Check sheet for the modelled part. Datum: model origin and axes. Units: mm. A direction names the side the tool comes from. Round coordinates to 2 decimals unless told otherwise and drop trailing zeros. Write each loop counter-clockwise with the first axis right and the second up, starting at its lowest first coordinate (ties: lowest second). Pieces come first, ordered by that corner, then holes. Notation, with made-up numbers: (29, 5.5) -> (78, 5.5) arc R16 cw to (78, 22.5) -> close; hole circle Ø3 at (71, 62). An arc over 180 degrees is marked (long way). Write item = value, one per line.
from build123d import *

# Parameters (mm, degrees)
SKETCH2_W                      = 50
SKETCH2_H                      = 50
BOSS_EXTRUDE1_DEPTH            = 10
SKETCH3_W                      = 9
SKETCH3_H                      = 9
CUT_EXTRUDE1_DEPTH             = 10
SKETCH4_R                      = 23.125
CUT_EXTRUDE2_DEPTH             = 2.5
F_4_0MM_DOWEL_HOLE1_D          = 4
FILLET1_R                      = 1
FILLET2_R                      = 10
CUT_EXTRUDE3_DEPTH             = 2.5
CBORE_FOR_M3_SHCS2_D           = 3.4
CBORE_FOR_M3_SHCS2_CBORE_D     = 6.5
CBORE_FOR_M3_SHCS2_CBORE_DEPTH = 3
SKETCH21_R                     = 3.25
CUT_EXTRUDE5_DEPTH             = 2.5
BOSS_EXTRUDE2_DEPTH            = 8
CHAMFER1_SIZE                  = 0.5


with BuildPart() as part:
    # Sketch2 → Boss-Extrude1 (new body)
    with BuildSketch(Plane(origin=(0, 0, 0), x_dir=(1, 0, 0), z_dir=(0, 1, 0))):
        Rectangle(SKETCH2_W, SKETCH2_H)
    extrude(amount=BOSS_EXTRUDE1_DEPTH)

    # Sketch3 → Cut-Extrude1 (cut)
    with BuildSketch(Plane(origin=(0, 10, 0), x_dir=(1, 0, 0), z_dir=(0, 1, 0))):
        Rectangle(SKETCH3_W, SKETCH3_H)
    extrude(amount=-CUT_EXTRUDE1_DEPTH, mode=Mode.SUBTRACT)

    # Sketch4 → Cut-Extrude2 (cut)
    with BuildSketch(Plane.XZ):
        Circle(SKETCH4_R)
    extrude(amount=-CUT_EXTRUDE2_DEPTH, mode=Mode.SUBTRACT)

    # Ø4.0mm Dowel Hole1 (through all)
    with Locations(Plane(origin=(0, 10, 0), x_dir=(1, 0, 0), z_dir=(0, 1, 0))):
        with Locations((-9, 5.5), (9, 5.5), (9, -5.5), (-9, -5.5)):
            Hole(F_4_0MM_DOWEL_HOLE1_D / 2)

    # Fillet1
    fillet1_edges = [part.edges().sort_by_distance(p)[0] for p in [
        (4.5, 6.25, -4.5),
        (-4.5, 6.25, -4.5),
        (-4.5, 6.25, 4.5),
        (4.5, 6.25, 4.5),
    ]]
    fillet(fillet1_edges, radius=FILLET1_R)

    # Fillet2
    fillet2_edges = [part.edges().sort_by_distance(p)[0] for p in [
        (-25, 5, -25),
        (25, 5, -25),
        (25, 5, 25),
        (-25, 5, 25),
    ]]
    fillet(fillet2_edges, radius=FILLET2_R)

    # Sketch17 → Cut-Extrude3 (cut)
    with BuildSketch(Plane(origin=(0, 10, 0), x_dir=(1, 0, 0), z_dir=(0, 1, 0))):
        with BuildLine():
            Line((5, 7.75), (11.25, 7.75))
            Line((11.25, 7.75), (11.25, -20.75))
            Line((11.25, -20.75), (-11.25, -20.75))
            Line((-11.25, -20.75), (-11.25, 7.75))
            Line((-11.25, 7.75), (-5, 7.75))
            ThreePointArc((-5, 7.75), (0, 12.75), (5, 7.75))
        make_face()
    extrude(amount=-CUT_EXTRUDE3_DEPTH, mode=Mode.SUBTRACT)

    # CBORE for M3 SHCS2 (through all)
    with Locations(Plane(origin=(0, 7.5, 0), x_dir=(1, 0, 0), z_dir=(0, 1, 0))):
        with Locations((0, -9), (0, 9)):
            CounterBoreHole(CBORE_FOR_M3_SHCS2_D / 2, CBORE_FOR_M3_SHCS2_CBORE_D / 2, CBORE_FOR_M3_SHCS2_CBORE_DEPTH)

    # Sketch21 → Cut-Extrude5 (cut)
    with BuildSketch(Plane(origin=(0, 10, 0), x_dir=(1, 0, 0), z_dir=(0, 1, 0))):
        with Locations((-9, 5.5)):
            Circle(SKETCH21_R)
        with Locations((9, 5.5)):
            Circle(SKETCH21_R)
        with Locations((9, -5.5)):
            Circle(SKETCH21_R)
        with Locations((-9, -5.5)):
            Circle(SKETCH21_R)
    extrude(amount=-CUT_EXTRUDE5_DEPTH, mode=Mode.SUBTRACT)

    # Sketch22 → Boss-Extrude2 (add)
    with BuildSketch(Plane(origin=(0, 10, 0), x_dir=(1, 0, 0), z_dir=(0, 1, 0))):
        with BuildLine():
            Line((-15, -25), (15, -25))
            ThreePointArc((15, -25), (22.071067812, -22.071067812), (25, -15))
            Line((25, -15), (25, 15))
            ThreePointArc((25, 15), (22.071067812, 22.071067812), (15, 25))
            Line((15, 25), (-15, 25))
            ThreePointArc((-15, 25), (-22.071067812, 22.071067812), (-25, 15))
            Line((-25, 15), (-25, -15))
            ThreePointArc((-25, -15), (-22.071067812, -22.071067812), (-15, -25))
        make_face()
        with BuildLine():
            Line((-11.25, 3.15479212), (-11.25, -3.15479212))
            ThreePointArc((-11.25, -3.15479212), (-12.25, -5.5), (-11.25, -7.84520788))
            Line((-11.25, -7.84520788), (-11.25, -20.75))
            Line((-11.25, -20.75), (11.25, -20.75))
            Line((11.25, -20.75), (11.25, -7.84520788))
            ThreePointArc((11.25, -7.84520788), (12.25, -5.5), (11.25, -3.15479212))
            Line((11.25, -3.15479212), (11.25, 3.15479212))
            ThreePointArc((11.25, 3.15479212), (11.298097039, 7.798097039), (6.65479212, 7.75))
            Line((6.65479212, 7.75), (5, 7.75))
            ThreePointArc((5, 7.75), (0, 12.75), (-5, 7.75))
            Line((-5, 7.75), (-6.65479212, 7.75))
            ThreePointArc((-6.65479212, 7.75), (-11.298097039, 7.798097039), (-11.25, 3.15479212))
        make_face(mode=Mode.SUBTRACT)
    extrude(amount=BOSS_EXTRUDE2_DEPTH)

    # Chamfer1
    chamfer1_edges = [part.edges().sort_by_distance(p)[0] for p in [
        (-22.071067812, 18, 22.071067812),
        (0, 18, 25),
        (22.071067812, 18, 22.071067812),
        (25, 18, 0),
        (22.071067812, 18, -22.071067812),
        (0, 18, -25),
        (-22.071067812, 18, -22.071067812),
        (-25, 18, 0),
        (-11.298097039, 18, -7.798097039),
        (-11.25, 18, 0),
        (-12.25, 18, 5.5),
        (-11.25, 18, 14.29760394),
        (0, 18, 20.75),
        (11.25, 18, 14.29760394),
        (12.25, 18, 5.5),
        (11.25, 18, 0),
        (11.298097039, 18, -7.798097039),
        (5.82739606, 18, -7.75),
        (0, 18, -12.75),
        (-5.82739606, 18, -7.75),
    ]]
    chamfer(chamfer1_edges, length=CHAMFER1_SIZE)


solid = part.part
(1) Access from +Z, -Z, +X, -X, +Y, -Y to the whole of each face (thin tool, end or side, straight path). Record for faces 1 (the cylindrical face through (0.37, 3.49, 10.66)), 2 (the flat face through (0, 12, 20.75)), 3 (the cylindrical face through (12.43, 1.23, 19.5)).
Worked answers:
face_1 = +Y, -Y
face_2 = +Y
face_3 = -Y
(2) Go/stop test with flat-tipped pins: P1, Ø2, axis at x = -1.5, z = 9.5, coming from the +Y side; P2, Ø6, axis at y = 5.5, z = 15.5, coming from the +X side; P3, Ø6, axis at x = 0, z = -9, coming from the -Y side; P4, Ø2, axis at x = 0, z = -9, coming from the +Y side. Record where each tip stops, or that it passes through.
Worked answers:
P1 = 4.5
P2 = 25
P3 = 2.5
P4 = through
(3) Sectioned sample at A-A on y = 14. Enter the section's corners in (x, z).
Worked answers:
outline = (-25, -15) arc R10 ccw to (-15, -25) -> (15, -25) arc R10 ccw to (25, -15) -> (25, 15) arc R10 ccw to (15, 25) -> (-15, 25) arc R10 ccw to (-25, 15) -> close; hole (-11.25, -3.15) arc R3.25 ccw (long way) to (-6.65, -7.75) -> (-5, -7.75) arc R5 ccw to (5, -7.75) -> (6.65, -7.75) arc R3.25 ccw (long way) to (11.25, -3.15) -> (11.25, 3.15) arc R3.25 ccw to (11.25, 7.85) -> (11.25, 20.75) -> (-11.25, 20.75) -> (-11.25, 7.85) arc R3.25 ccw to (-11.25, 3.15) -> close
(4) Sectioned sample at D-D on z = 2. Enter the section's corners in (x, y).
Worked answers:
outline = (-25, 0) -> (-23.04, 0) -> (-23.04, 2.5) -> (-4.5, 2.5) -> (-4.5, 7.5) -> (-11.25, 7.5) -> (-11.25, 17.5) -> (-11.75, 18) -> (-24.5, 18) -> (-25, 17.5) -> close; (4.5, 2.5) -> (23.04, 2.5) -> (23.04, 0) -> (25, 0) -> (25, 17.5) -> (24.5, 18) -> (11.75, 18) -> (11.25, 17.5) -> (11.25, 7.5) -> (4.5, 7.5) -> close
(5) Material ranges on L1, parallel to Z at x = 9, y = 4.7; L2, parallel to Z at x = 0, y = 5.95; L3, parallel to X at y = 14, z = 13, recorded low to high. Write a range as [from, to].
Worked answers:
L1 = [-25, -7.5], [-3.5, 3.5], [7.5, 25]
L2 = [-25, -12.25], [-5.75, -4.5], [4.5, 5.75], [12.25, 25]
L3 = [-25, -11.25], [11.25, 25]
(6) Sectioned sample at C-C on y = 3.25. Enter the section's corners in (x, z).
Worked answers:
outline = (-25, -15) arc R10 ccw to (-15, -25) -> (15, -25) arc R10 ccw to (25, -15) -> (25, 15) arc R10 ccw to (15, 25) -> (-15, 25) arc R10 ccw to (-25, 15) -> close; hole circle Ø4 at (-9, -5.5); hole circle Ø4 at (-9, 5.5); hole (-4.5, -3.5) arc R1 ccw to (-3.5, -4.5) -> (3.5, -4.5) arc R1 ccw to (4.5, -3.5) -> (4.5, 3.5) arc R1 ccw to (3.5, 4.5) -> (-3.5, 4.5) arc R1 ccw to (-4.5, 3.5) -> close; hole circle Ø3.4 at (0, -9); hole circle Ø3.4 at (0, 9); hole circle Ø4 at (9, -5.5); hole circle Ø4 at (9, 5.5)
(7) Release check for a two-part mould opening along Z. For faces 4 (the conical face through (-21.89, 17.86, 21.74)), 5 (the flat face through (25, 9, 0)), 6 (the flat face through (11.25, 12, 0)) record: pulls with the +Z half, pulls with the -Z half, needs draft (parallel to the pull), parting line crosses it, or undercut.
Worked answers:
face_4 = pulls with the +Z half
face_5 = needs draft
face_6 = undercut
(8) Sectioned sample at B-B on x = -9. Enter the section's corners in (y, z).
Worked answers:
outline = (0, -25) -> (17.5, -25) -> (18, -24.5) -> (18, -9.25) -> (17.5, -8.75) -> (7.5, -8.75) -> (7.5, -7.5) -> (2.5, -7.5) -> (2.5, -21.3) -> (0, -21.3) -> close; (0, 21.3) -> (2.5, 21.3) -> (2.5, 7.5) -> (7.5, 7.5) -> (7.5, 20.75) -> (17.5, 20.75) -> (18, 21.25) -> (18, 24.5) -> (17.5, 25) -> (0, 25) -> close; (2.5, -3.5) -> (7.5, -3.5) -> (7.5, 3.5) -> (2.5, 3.5) -> close
